Part model, mm, in its own coordinate system. A direction names the side the tool comes from. Give positions to 0.01 mm unless a question says otherwise; leave off trailing zeros. Write each loop counter-clockwise with the first axis right and the second up, starting at its lowest first coordinate (ties: lowest second). Pieces come first, ordered by that corner, then holes.
Autodesk Inventor part; units mm, degrees
ref_plane "YZ Plane" through (0, 0, 0) normal (1, 0, 0) x (0, 1, 0)
ref_plane "XZ Plane" through (0, 0, 0) normal (0, 1, 0) x (-1, 0, 0)
ref_plane "XY Plane" through (0, 0, 0) normal (0, 0, 1) x (1, 0, 0)
sketch "Sketch1" plane through (0, 0, 0) normal (0, 0, 1) x (1, 0, 0)
  line L0 (0, 0) -> (0, 34)
  line L1 (0, 34) -> (18, 34)
  line L2 (18, 34) -> (18, 0)
  line L3 (18, 0) -> (18, 21)
  line L4 (18, 21) -> (39, 21)
  line L5 (39, 21) -> (39, 0)
  line L6 (39, 0) -> (39, 15)
  line L7 (39, 15) -> (50, 15)
  line L8 (50, 15) -> (50, 0)
  line L9 (50, 0) -> (50, 10)
  line L10 (50, 10) -> (60, 10)
  line L11 (60, 10) -> (60, 0)
  line L12 (60, 0) -> (60, 8)
  line L13 (60, 8) -> (74, 8)
  line L14 (74, 8) -> (74, 0)
  line L15 (0, 0) -> (74, 0)
  line L16 (0, 0) -> (84.2736, 0) construction
  dimension "d0" = 34
  dimension "d1" = 18
  dimension "d2" = 34
  dimension "d3" = 21
  dimension "d4" = 21
  dimension "d5" = 15
  dimension "d6" = 11
  dimension "d7" = 10
  dimension "d9" = 10
  dimension "d10" = 8
  dimension "d11" = 14
revolve "Revolution1" add sketch "Sketch1" angle 360 about axis through (0, 0, 0) along (1, 0, 0)
properties part number "5 Cilindros centrales" material "Aluminum 6061"
1) Pin check, flat tips, straight feed: pin 1 Ø5 at (x, y) = (15.5, 24) entering from -Z; pin 2 Ø1 at (x, y) = (51.5, -11) entering from -Z; pin 3 Ø5 at (x, z) = (9.5, -18.5) entering from -Y; pin 4 Ø5 at (y, z) = (-11, -23) entering from +X. Stop position of each tip, or through.
Answers follow:
pin 1: stops at z = -26.34
pin 2: passes through
pin 3: stops at y = -30
pin 4: stops at x = 18
2) Saw through at A-A, the plane z = 7. Write the cut outline in (x, y).
Answers follow:
outline: (0, -33.27) - (18, -33.27) - (18, -19.8) - (39, -19.8) - (39, -13.27) - (50, -13.27) - (50, -7.14) - (60, -7.14) - (60, -3.87) - (74, -3.87) - (74, 3.87) - (60, 3.87) - (60, 7.14) - (50, 7.14) - (50, 13.27) - (39, 13.27) - (39, 19.8) - (18, 19.8) - (18, 33.27) - (0, 33.27) - close
3) Wall check: L1, parallel to X at y = 25.5, z = -21.5; L2, parallel to Z at x = 68, y = -0.5; L3, parallel to X at y = 15, z = 7.5. Give the ranges that are in metal, low to high.
Answers follow:
L1: x = 0 to 18
L2: z = -7.98 to 7.98
L3: x = 0 to 39
4) Saw through at B-B, the plane y = 0. Write the cut outline in (x, z), then the cut area to 3 significant figures.
Answers follow:
outline: (0, -34) - (18, -34) - (18, -21) - (39, -21) - (39, -15) - (50, -15) - (50, -10) - (60, -10) - (60, -8) - (74, -8) - (74, 8) - (60, 8) - (60, 10) - (50, 10) - (50, 15) - (39, 15) - (39, 21) - (18, 21) - (18, 34) - (0, 34) - close
area: 2,860 mm2
5) Saw through at D-D, the plane z = -12.5. Write the cut outline in (x, y).
Answers follow:
outline: (0, -31.62) - (18, -31.62) - (18, -16.87) - (39, -16.87) - (39, -8.29) - (50, -8.29) - (50, 8.29) - (39, 8.29) - (39, 16.87) - (18, 16.87) - (18, 31.62) - (0, 31.62) - close
6) 3-axis set-ups, long thin cutter, end or side, ignore diameter. For faces 1 (the face through (67.1, -1.73, -7.81)), 2 (the face through (74, 0, 0)): which of +Z, -Z, +X, -X, +Y, -Y reach the whole face in a straight line?
Answers follow:
face 1: +X
face 2: +Z, -Z, +X, +Y, -Y
7) Saw through at C-C, the plane x = 41. Write the cut outline in (y, z), then the cut area to 3 significant figures.
Answers follow:
outline: circle Ø30 at (0, 0)
area: 707 mm2
